from build123d import *

# Parameters (mm, degrees)
SKETCH4_W           = 19.05
SKETCH4_H           = 19.05
SKETCH4_W_2         = 15.24
SKETCH4_H_2         = 15.24
BOSS_EXTRUDE2_DEPTH = 457.2
CUT_EXTRUDE1_DEPTH  = 20.05


with BuildPart() as part:
    # Sketch4 → Boss-Extrude2 (new body)
    with BuildSketch(Plane.XY):
        Rectangle(SKETCH4_W, SKETCH4_H)
        Rectangle(SKETCH4_W_2, SKETCH4_H_2, mode=Mode.SUBTRACT)
    extrude(amount=BOSS_EXTRUDE2_DEPTH)

    # Sketch5 → Cut-Extrude1 (cut, through all)
    with BuildSketch(Plane(origin=(9.525, 0, 0), x_dir=(0, 0, -1), z_dir=(1, 0, 0))):
        Polygon((-457.2, 9.525), (-448.316839112, -9.525), (-457.2, -9.525), align=None)
    extrude(amount=-CUT_EXTRUDE1_DEPTH, mode=Mode.SUBTRACT)


solid = part.part
The listing builds one solid part. Answer for the finished solid, in the listing's coordinates (mm). A direction names the side the tool comes from. Give positions to 0.01 mm unless a question says otherwise; leave off trailing zeros. Write each loop counter-clockwise with the first axis right and the second up, starting at its lowest first coordinate (ties: lowest second). Pieces come first, ordered by that corner, then holes. Notation, with made-up numbers: (-9, -15) - (45, -15) arc R25 cw to (45, 3) - close; hole circle Ø11 at (2.25, 66.25). An arc over 180 degrees is marked (long way). Use a Markdown table: item, result.
1. Section A-A on x = -4 is taken. Write down the section's boundary in (y, z) (3 decimals), plus the area to 3 significant figures.
Values follow:
| item | result |
|---|---|
| outline | (-9.525, 0) - (-7.62, 0) - (-7.62, 449.205) - (-9.525, 448.317) - close; (7.62, 0) - (9.525, 0) - (9.525, 457.2) - (7.62, 456.312) - close |
| area | 1,730 mm² |
2. Section B-B on z = 258 is taken. Write down the section's boundary in (x, y) (3 decimals).
Values follow:
| item | result |
|---|---|
| outline | (-9.525, -9.525) - (9.525, -9.525) - (9.525, 9.525) - (-9.525, 9.525) - close; hole (-7.62, -7.62) - (7.62, -7.62) - (7.62, 7.62) - (-7.62, 7.62) - close |
3. Section C-C on y = -0.25 is taken. Write down the section's boundary in (x, z) (3 decimals), plus the area to 3 significant figures.
Values follow:
| item | result |
|---|---|
| outline | (-9.525, 0) - (-7.62, 0) - (-7.62, 452.642) - (-9.525, 452.642) - close; (7.62, 0) - (9.525, 0) - (9.525, 452.642) - (7.62, 452.642) - close |
| area | 1,720 mm² |
4. For a pull along Y with two mould halves and no side action, classify faces 1 (the flat face through (-7.62, 0, 225)), 2 (the flat face through (9.525, 0, 225)), 3 (the flat face through (0, -9.525, 221)) as released by +Y, released by -Y, zero draft, split by the parting line, or undercut.
Values follow:
| item | result |
|---|---|
| face 1 | undercut |
| face 2 | zero draft |
| face 3 | released by -Y |
5. This flat-tipped pin is pushed along its axis until it touches: P1, Ø10, axis at x = -4, y = 6, coming from the +Z side. Where does it stop, or does it pass through?
Values follow:
| item | result |
|---|---|
| P1 | stops at z = 457.2 |
6. Find the intervals of material crossed by probe 1 along X at (y, z) = (-2.75, 99) (3 decimals); probe 2 along Z at (x, y) = (1.5, 7.75), in increasing order. Write a range as from..to.
Values follow:
| item | result |
|---|---|
| probe 1 | x = -9.525..-7.62, 7.62..9.525 |
| probe 2 | z = 0..456.37 |
7. A tool of negligible diameter and unlimited length cuts with its end or side. For faces 4 (the flat face through (-9, 0, 0)), 5 (the flat face through (7.62, 0, 225)), from which of +Z, -Z, +X, -X, +Y, -Y can it reach the whole face along a straight path? Write none if from no direction.
Values follow:
| item | result |
|---|---|
| face 4 | -Z, +X, -X, +Y, -Y |
| face 5 | +Z, -Z |
